Verification items for the finished model (mm, model axes). Face numbers are marked on the shaded views. Give positions to 0.01 mm unless a question says otherwise; leave off trailing zeros. Write each loop counter-clockwise with the first axis right and the second up, starting at its lowest first coordinate (ties: lowest second). Pieces come first, ordered by that corner, then holes. Notation, with made-up numbers: (69, 78.25) - (111, 78.25) arc R15 ccw to (111, 97.25) - close; hole circle Ø11 at (75, 44.5). An arc over 180 degrees is marked (long way). Answer as a JSON object with one key per item and string values. Group by question number.
Item 1: Sectioned sample at D-D, the plane z = -38.5. Record the boundary of the cut face in (x, y), and give its area (3 significant figures).
Item 2: Sectioned sample at B-B, the plane x = -47. Record the boundary of the cut face in (y, z).
Item 3: Sectioned sample at A-A, the plane z = 11. Record the boundary of the cut face in (x, y), and give its area (3 significant figures).
Item 4: Draft check along Z on the marked faces 1 and 2. Enter one of: +Z half, -Z half, draft (parallel to the pull), parting line (faces both ways), or undercut.
Item 5: Sectioned sample at C-C, the plane z = -6.5. Record the boundary of the cut face in (x, y).
Item 6: Go/stop test with flat-tipped pins: pin 1 (12 mm diameter, centred on y = 35, z = -28.5, fed in from +X); pin 2 (1.5 mm diameter, centred on x = -20.5, z = -6, fed in from +Y); pin 3 (1 mm diameter, centred on x = -21.5, z = 0.5, fed in from -Y). Record where each tip stops, or that it passes through.
Item 7: Scan lines: line 1 along Y through (x, z) = (1, 19.5); line 2 along Y through (x, z) = (-43, 24); line 3 along X through (y, z) = (46.5, -38.5). Record each from-to range of solid material in increasing order. Write a range as [from, to].
```python
from build123d import *

# Parameters (mm, degrees)
BOSS_EXTRUDE1_DEPTH = 50
CUT_EXTRUDE1_DEPTH  = 10
SKETCH3_R           = 4
CUT_EXTRUDE2_DEPTH  = 10
SKETCH4_W           = 1.052304973
SKETCH4_H           = 5.165860775
CUT_EXTRUDE6_DEPTH  = 0.5
CUT_EXTRUDE7_DEPTH  = 2
SKETCH6_R           = 0.804992829
SKETCH6_R_2         = 0.803708801
BOSS_EXTRUDE2_DEPTH = 3


with BuildPart() as part:
    # Sketch1 → Boss-Extrude1 (new, symmetric)
    with BuildSketch(Plane.XY):
        Polygon((0, 0), (4.242640687, 0), (-45.757359313, 50), (-50, 50), align=None)
    extrude(amount=BOSS_EXTRUDE1_DEPTH, both=True)

    # Sketch2 → Cut-Extrude1 (cut)
    with BuildSketch(Plane(origin=(2.121320344, 2.121320344, 0), x_dir=(0, 0, -1), z_dir=(0.7071067811865487, 0.7071067811865465, 0))):
        with BuildLine():
            Line((-32.383146044, 21.19659939), (-17.279022802, 21.19659939))
            Line((-17.279022802, 21.19659939), (-14.530403118, 28.687350871))
            ThreePointArc((-14.530403118, 28.687350871), (-25.009728549, 61.996596804), (-35.453632693, 28.676227773))
            Line((-35.453632693, 28.676227773), (-32.383146044, 21.19659939))
        make_face()
    extrude(amount=-CUT_EXTRUDE1_DEPTH, mode=Mode.SUBTRACT)

    # Sketch3 → Cut-Extrude2 (cut)
    with BuildSketch(Plane(origin=(2.121320344, 2.121320344, 0), x_dir=(0, 0, -1), z_dir=(0.7071067811865487, 0.7071067811865465, 0))):
        with Locations(Location((29.848579643, 15.751722073, 0), (0, 0, 90))):
            Circle(SKETCH3_R)
    extrude(amount=-CUT_EXTRUDE2_DEPTH, mode=Mode.SUBTRACT)

    # Sketch4 → Cut-Extrude6 (cut)
    with BuildSketch(Plane(origin=(2.121320344, 2.121320344, 0), x_dir=(0, 0, -1), z_dir=(0.7071067811865488, 0.7071067811865462, 0))):
        Polygon((18.209716016, 48.632673253), (18.209716016, 42.984750661), (23.10096046, 45.808711957), align=None)
        with Locations((23.211533522, 45.906886197)):
            Rectangle(SKETCH4_W, SKETCH4_H)
        with Locations((25.236963378, 45.906886197)):
            Rectangle(SKETCH4_W, SKETCH4_H)
        Polygon((32.568799155, 48.489816584), (32.568799155, 43.12760733), (37.212608589, 45.808711957), align=None)
        Polygon((36.890986923, 48.489816584), (36.890986923, 43.12760733), (41.534796358, 45.808711957), align=None)
        Polygon((9.151606642, 48.632673253), (9.151606642, 42.984750661), (4.260362198, 45.808711957), align=None)
        Polygon((4.590275544, 48.355357963), (4.590275544, 43.262065951), (0.179355272, 45.808711957), align=None)
    extrude(amount=-CUT_EXTRUDE6_DEPTH, mode=Mode.SUBTRACT)

    # Sketch5 → Cut-Extrude7 (cut)
    with BuildSketch(Plane(origin=(0, 0, 0), x_dir=(0, 0, 1), z_dir=(-0.7071067811865488, -0.7071067811865462, 0))):
        Polygon((46.201031171, 64.525111683), (46.201031171, 13.41528861), (3.998852775, 13.41528861), (3.998852775, 2.899934094), (-43.862101498, 2.899934094), (-43.862101498, 38.281153906), (-43.862101498, 54.027620673), (3.998852775, 54.027620673), (3.998852775, 64.525111683), align=None)
    extrude(amount=-CUT_EXTRUDE7_DEPTH, mode=Mode.SUBTRACT)

    # Sketch6 → Boss-Extrude2 (add)
    with BuildSketch(Plane(origin=(2.121320344, 2.121320344, 0), x_dir=(0, 0, -1), z_dir=(0.7071067811865488, 0.7071067811865462, 0))):
        with Locations(Location((-34.35, 21.73, 0), (0, 0, 90))):
            Circle(SKETCH6_R)
        with Locations(Location((-15.49, 21.73, 0), (0, 0, 90))):
            Circle(SKETCH6_R_2)
    extrude(amount=-BOSS_EXTRUDE2_DEPTH)


solid = part.part
```
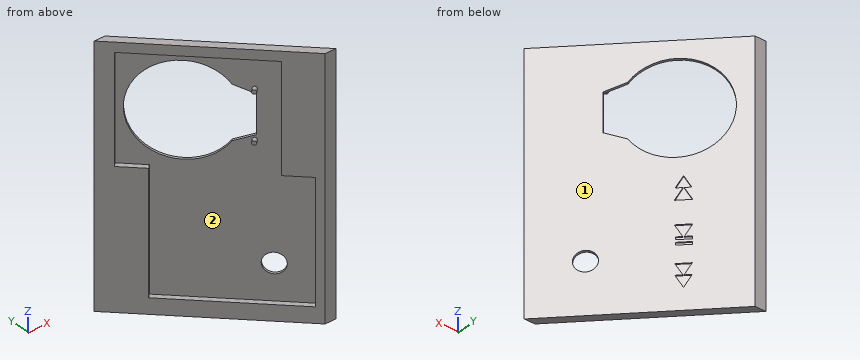
Geometry check:
{
 "1": {"outline": "(-50, 50) - (-38.2, 38.2) - (-36.79, 39.62) - (-0.64, 3.46) - (-2.05, 2.05) - (0, 0) - (4.24, 0) - (-29.03, 33.27) - (-29.38, 32.92) - (-31.86, 35.4) - (-31.51, 35.75) - (-45.76, 50) - close", "area": "108 mm^2"},
 "2": {"outline": "(47, -50) - (50, -50) - (50, 50) - (47, 50) - close"},
 "3": {"outline": "(-50, 50) - (-45.63, 45.63) - (-44.21, 47.04) - (-37.82, 40.65) - (-37.11, 41.35) - (-45.76, 50) - close; (-21.15, 23.98) - (-8.07, 10.9) - (-9.49, 9.49) - (0, 0) - (4.24, 0) - (-20.44, 24.69) - close", "area": "86.3 mm^2"},
 "4": {"face 1": "draft", "face 2": "undercut"},
 "5": {"outline": "(-50, 50) - (-38.2, 38.2) - (-36.79, 39.62) - (-0.64, 3.46) - (-2.05, 2.05) - (0, 0) - (4.24, 0) - (-29.36, 33.6) - (-29.71, 33.25) - (-31.54, 35.07) - (-31.18, 35.43) - (-45.76, 50) - close"},
 "6": {"pin 1": "x = -24.76", "pin 2": "y = 25.49", "pin 3": "y = 23.83"},
 "7": {"line 1": "[0, 3.24]", "line 2": "[45.83, 47.24]", "line 3": "[-46.5, -42.26]"}
}
